The model under review builds one solid part; all positions refer to its coordinate system, in mm. A direction names the side the tool comes from. Coordinates: 2 decimals unless noted, no trailing zeros. Order: outer loops, then holes, each group sorted by start corner. A loop starts at its lowest first (then second) coordinate and runs counter-clockwise, first axis right, second up.
Autodesk Inventor part; units mm, degrees
ref_plane "YZ Plane" through (0, 0, 0) normal (1, 0, 0) x (0, 1, 0)
ref_plane "XZ Plane" through (0, 0, 0) normal (0, 1, 0) x (-1, 0, 0)
ref_plane "XY Plane" through (0, 0, 0) normal (0, 0, 1) x (1, 0, 0)
sketch "Sketch1" plane through (0, 0, 0) normal (0, 1, 0) x (-1, 0, 0)
  circle A0 centre (0, 0) radius 2.5
  dimension "d0" = 5
extrude "Extrusion1" add sketch "Sketch1" along normal blind 5
chamfer "Chamfer1" distance 1 angle 45 1 edges at (2.5, 0, 0)
sketch "Sketch2" plane through (0, 5, 0) normal (0, 1, 0) x (1, 0, 0)
  point P0 (0, 0)
  point P1 (0, 0)
hole "Hole1" at (0, 5, 0) direction (0, -1, 0) diameter 2.459 depth 3
properties part number "Insert" material "Brass, Soft Yellow"
(1) Consider section C-C (y = 2.2). Give the boundary of the cut face in (x, z).
(2) Consider section A-A (x = 0). Give the boundary of the cut face in (y, z), then the cut area to 3 significant figures.
(3) The part is to be moulded in two halves that separate along Z. For faces 1 (the face through (0.54, 2.97, 2.44)), 2 (the face through (0.748, 3.479, -0.976)), 3 (the face through (0, 0, 0)), say which applies: +Z half, -Z half, draft (parallel to the pull), parting line (faces both ways), or undercut.
(4) Consider section B-B (z = 0). Give the boundary of the cut face in (x, y), then the cut area to 3 significant figures.
(5) Insertion check: pin 1 Ø1.5 at (x, z) = (0, 0) entering from -Y; pin 2 Ø1 at (y, z) = (1.5, -1) entering from +X; pin 3 Ø0.7 at (x, z) = (-0.5, 0.5) entering from +Y. Each pin has a flat end and moves straight along its axis. Give the tip position at first contact, or say it passes through.
(6) Consider section D-D (y = 0.6). Give the boundary of the cut face in (x, z).
(7) Wall thickness on line 1 (Z direction, x = 0, y = 3.35); line 2 (Y direction, x = -0.2, z = -0.25); line 3 (X direction, y = 3.6, z = -0.8): over which ranges is each line inside the solid? List them lowest first.
(8) Tool access review of faces 4 (the face through (-1, 5, 1)), 5 (the face through (0, 2, 0)): name each direction out of +Z, -Z, +X, -X, +Y, -Y from which nothing blocks a thin tool from reaching the whole face with its end or side.
Findings:
1. outline: circle Ø5 at (0, 0); hole circle Ø2.46 at (0, 0)
2. outline: (0, -1.5) - (1, -2.5) - (5, -2.5) - (5, -1.23) - (2, -1.23) - (2, 1.23) - (5, 1.23) - (5, 2.5) - (1, 2.5) - (0, 1.5) - close
2. area: 16.6 mm2
3. face 1: parting line
3. face 2: undercut
3. face 3: draft
4. outline: (-2.5, 1) - (-1.5, 0) - (1.5, 0) - (2.5, 1) - (2.5, 5) - (1.23, 5) - (1.23, 2) - (-1.23, 2) - (-1.23, 5) - (-2.5, 5) - close
4. area: 16.6 mm2
5. pin 1: stops at y = 0
5. pin 2: stops at x = 2.45
5. pin 3: stops at y = 2
6. outline: circle Ø4.2 at (0, 0)
7. line 1: z = -2.5 to -1.23, 1.23 to 2.5
7. line 2: y = 0 to 2
7. line 3: x = -2.37 to -0.93, 0.93 to 2.37
8. face 4: +Z, -Z, +X, -X, +Y
8. face 5: +Y
